Build history of the part. All positions in model axes, mm. Give positions to 0.01 mm unless a question says otherwise; leave off trailing zeros. Loops run counter-clockwise (first coordinate to the right, second up) from the corner with the lowest first, then second, coordinate; pieces in that order, holes last. Notation, with made-up numbers: (53.5, 44) - (93.5, 44) arc R20 cw to (93.5, 49) - close; hole circle Ø4 at (16, 46). An arc over 180 degrees is marked (long way). Return JSON: item names as keys, results as strings. Group by question number.
1) Slice it at A-A (z = -12). List the corners of the cut face in (x, y).
2) Drop a flat-ended pin along its axis: pin 1 (2.5 mm diameter, centred on x = 0, z = 18.5, fed in from +Y). Give the stop position or say it passes through.
3) Drill centre lines: probe 1 along Y at (x, z) = (1.5, 26); probe 2 along X at (y, z) = (0.25, -3.5); probe 3 along X at (y, z) = (-2.2, 8). Where is each one in solid material? Low to high. Write a range as from..to.
4) Mould opens along Z. For faces 1 (the face through (0, 0, -29.75)), 2 (the face through (0, 0, 29.75)), 3 (the face through (0.33, -2.48, 0.41)) say: released by +Z, released by -Z, zero draft, split by the parting line, or undercut.
5) Slice it at B-B (z = 10.5). List the corners of the cut face in (x, y).
```python
from build123d import *

# Parameters (mm, degrees)
SKETCH1_R           = 2.5
BOSS_EXTRUDE1_DEPTH = 29.75
CUT_EXTRUDE2_DEPTH  = 20
FILLET1_R           = 0.5


with BuildPart() as part:
    # Sketch1 → Boss-Extrude1 (new, symmetric)
    with BuildSketch(Plane.XY):
        with Locations(Location((0, 0, 0), (0, 0, 180))):
            Circle(SKETCH1_R)
    extrude(amount=BOSS_EXTRUDE1_DEPTH, both=True)

    # Sketch2 → Cut-Extrude2 (cut)
    with BuildSketch(Plane.XY.offset(29.75)):
        with BuildLine():
            ThreePointArc((1.5, 2), (0, 2.5), (-1.5, 2))
            Line((-1.5, 2), (1.5, 2))
        make_face()
    extrude(amount=-CUT_EXTRUDE2_DEPTH, mode=Mode.SUBTRACT)

    # Fillet1
    fillet1_edges = [part.edges().sort_by_distance(p)[0] for p in [
        (2.5, 0, -29.75),
        (1.118033989, -2.236067977, 29.75),
    ]]
    fillet(fillet1_edges, radius=FILLET1_R - 0.0001)  # a hair under: the kernel refuses the full size


solid = part.part
```
Results:
{
 "1": {"outline": "circle Ø5 at (0, 0)"},
 "2": {"pin 1": "y = 2"},
 "3": {"probe 1": "-2..2", "probe 2": "-2.49..2.49", "probe 3": "-1.19..1.19"},
 "4": {"face 1": "released by -Z", "face 2": "released by +Z", "face 3": "zero draft"},
 "5": {"outline": "(-1.5, 2) arc R2.5 ccw (long way) to (1.5, 2) - close"}
}
